Model file for the job. Use its own axes, mm. A direction names the side the tool comes from. Coordinates: 2 decimals unless noted, no trailing zeros. Write each loop counter-clockwise with the first axis right and the second up, starting at its lowest first coordinate (ties: lowest second). Pieces come first, ordered by that corner, then holes.
Q1. Which spindle directions (+Z, -Z, +X, -X, +Y, -Y) get a long thin tool onto all of the face, cutting with end or side? Do faces 1 (the cylindrical face through (33.499, 85.285, 2.861)), 2 (the cylindrical face through (36, 83.7, 2.4)), 3 (the cylindrical face through (1.025, 23.005, 7.808)). Say none if no direction does.
Q2. Band-saw the part on A-A, the plane z = 0. Write the cut outline in (x, y) (3 decimals).
Q3. Pull direction X, two halves, no side cores. Call faces 4 (the flat face through (41.1, 76.4, -8.1)), 5 (the conical face through (36.288, 86.764, 1.387)), 6 (the cylindrical face through (7.559, 23.005, -5.796)), 7 (the flat face through (7, 0, -4)): released by +X, released by -X, zero draft, split by the parting line, or undercut.
Q4. Pin check, flat tips, straight feed: P1, Ø2, axis at x = 29, z = 4, coming from the +Y side; P2, Ø1, axis at x = 32.5, z = -3, coming from the -Y side; P3, Ø4, axis at y = 27, z = -9.5, coming from the +X side; P4, Ø4, axis at y = 73.5, z = 6, coming from the +X side. Stop position of each tip, or through.
Q5. Drill centre lines: probe 1 along Z at (x, y) = (0, 23) (3 decimals); probe 2 along Z at (x, y) = (4.5, 25); probe 3 along Y at (x, z) = (35.25, 0) (3 decimals). Where is each one in solid material? Low to high.
Q6. Band-saw the part on B-B, the plane y = 10.5. Write the cut outline in (x, z) (3 decimals), plus the area to 3 significant figures.
Autodesk Inventor part; units mm, degrees
ref_plane "YZ Plane" through (0, 0, 0) normal (1, 0, 0) x (0, 1, 0)
ref_plane "XZ Plane" through (0, 0, 0) normal (0, 1, 0) x (-1, 0, 0)
ref_plane "XY Plane" through (0, 0, 0) normal (0, 0, 1) x (1, 0, 0)
sketch "Sketch1" plane through (0, 0, 0) normal (0, 0, 1) x (1, 0, 0)
  line L0 (0, 0) -> (0, 45.375)
  line L1 (30.825, 76.2) -> (41.1, 76.2)
  arc A0 (30.825, 76.2) -> (0, 45.375) centre (30.825, 45.375) ccw
  dimension "d1" = 76.2
  dimension "d2" = 41.1
  dimension "d4" = 30.825
sketch "Sketch2" plane through (0, 0, 0) normal (0, 1, 0) x (-1, 0, 0)
  circle A0 centre (0, 0) radius 9.525
  circle A1 centre (0, 0) radius 7.875
  dimension "d3" = 19.05
  dimension "d11" = 1.65
sweep "Sweep1" add profiles "Sketch2" path "Sketch1"
sketch "Sketch3" plane through (41.1, 76.2, 0) normal (1, 0, 0) x (0, 0, -1)
  circle A0 centre (0, 0) radius 9.525
  circle A1 centre (0, 0) radius 12.45
  point P0 (0, -76.2)
  dimension "d6" = 24.9
extrude "Extrusion1" add sketch "Sketch3" against normal blind 5
chamfer "Chamfer1" distance 3 distance2 1.9154 1 edges at (36.1, 76.2, 12.45) measured on face at (37.7667, 74.2029, -12.2888)
equation "\"d4\" = 0.75 * d2"
equation "\"d15\" = 0.0769231 * d6"
properties part number "Ferrule 90 deg Elb-19.05"
Answer sheet:
1. face 1: none
1. face 2: +X
1. face 3: -Y
2. outline: (-9.525, 0) - (-7.875, 0) - (-7.875, 45.375) arc R38.7 cw to (30.825, 84.075) - (41.1, 84.075) - (41.1, 88.65) - (39.1, 88.65) - (36.1, 86.735) - (36.1, 85.725) - (30.825, 85.725) arc R40.35 ccw to (-9.525, 45.375) - close; (7.875, 0) - (9.525, 0) - (9.525, 45.375) arc R21.3 cw to (30.825, 66.675) - (36.1, 66.675) - (36.1, 65.665) - (39.1, 63.75) - (41.1, 63.75) - (41.1, 68.325) - (30.825, 68.325) arc R22.95 ccw to (7.875, 45.375) - close
3. face 4: released by +X
3. face 5: undercut
3. face 6: split by the parting line
3. face 7: zero draft
4. P1: stops at y = 85.2
4. P2: stops at y = 67.01
4. P3: stops at x = 5.87
4. P4: stops at x = 41.1
5. probe 1: z = -9.525 to -7.875, 7.875 to 9.525
5. probe 2: z = -8.39 to -6.46, 6.46 to 8.39
5. probe 3: y = 66.675 to 68.325, 84.075 to 85.725
6. outline: circle Ø19.05 at (0, 0); hole circle Ø15.75 at (0, 0)
6. area: 90.2 mm2
